Could you check a few things on this model? Use its own coordinates, in mm. Face numbers are marked on the shaded views. A direction names the side the tool comes from. Round coordinates to 2 decimals unless told otherwise and drop trailing zeros. Loops run counter-clockwise (first coordinate to the right, second up) from the corner with the lowest first, then second, coordinate; pieces in that order, holes last.
from build123d import *

# Parameters (mm, degrees)
BOSS_EXTRUDE1_DEPTH = 6.5
BOSS_EXTRUDE2_START = 6.5
SKETCH1_4_R         = 7.5
SKETCH1_4_R_2       = 1.55
BOSS_EXTRUDE2_DEPTH = 9
CUT_EXTRUDE1_DEPTH  = 15
CHAMFER1_SIZE       = 5
FILLET1_R           = 1
CUT_EXTRUDE2_DEPTH  = 3


with BuildPart() as part:
    # Sketch1 → Boss-Extrude1 (new, symmetric)
    with BuildSketch(Plane(origin=(0, 0, 0), x_dir=(1, 0, 0), z_dir=(0, 1, 0))):
        with BuildLine():
            Line((-1, 0), (0, 0))
            Line((0, 0), (0, 16))
            Line((0, 16), (-16, 16))
            ThreePointArc((-16, 16), (-17.414213562, 15.414213562), (-18, 14))
            Line((-18, 14), (-18, -14))
            ThreePointArc((-18, -14), (-10.5, -6.5), (-3, -14))
            Line((-3, -14), (-3, -2))
            ThreePointArc((-3, -2), (-2.414213562, -0.585786438), (-1, 0))
        make_face()
    extrude(amount=BOSS_EXTRUDE1_DEPTH, both=True)

    # Sketch1<4> → Boss-Extrude2 (add)
    with BuildSketch(Plane(origin=(0, 0, 0), x_dir=(1, 0, 0), z_dir=(0, 1, 0)).offset(BOSS_EXTRUDE2_START)):
        with Locations((-10.5, -14)):
            Circle(SKETCH1_4_R)
        with Locations(Location((-10.5, -14, 0), (0, 0, 270))):
            Circle(SKETCH1_4_R_2, mode=Mode.SUBTRACT)
    extrude(amount=-BOSS_EXTRUDE2_DEPTH)

    # Sketch2 → Cut-Extrude1 (cut)
    with BuildSketch(Plane(origin=(0, 0, 0), x_dir=(0, 0, -1), z_dir=(1, 0, 0))):
        with BuildLine():
            ThreePointArc((12.5, 0), (9.505604778, 4.240654932), (4.507486999, 2.837666813))
            Line((4.507486999, 2.837666813), (11.492513001, -2.837666813))
            ThreePointArc((11.492513001, -2.837666813), (12.240654932, -1.505604778), (12.5, 0))
        make_face()
        with BuildLine():
            Line((11.492513001, -2.837666813), (4.507486999, 2.837666813))
            ThreePointArc((4.507486999, 2.837666813), (5.162333187, -3.492513001), (11.492513001, -2.837666813))
        make_face()
    extrude(amount=-CUT_EXTRUDE1_DEPTH, mode=Mode.SUBTRACT)

    # Chamfer1
    # the kernel refuses this chamfer: 5 mm, written as the material it takes off along each edge
    with BuildSketch(Plane(origin=(-10.5, -6.5, 14), x_dir=(-0.003141587485879666, 0, 0.9999950652018581), z_dir=(0.9999950652018581, 0, 0.003141587485879666))) as chamfer1_piece_1_section:
        Polygon((7.5 + CHAMFER1_SIZE, 0), (7.5, -CHAMFER1_SIZE), (7.5, 0), align=None)
    chamfer1_piece_1 = revolve(axis=Axis((-10.5, -6.5, 14), (0, -1, 0)), revolution_arc=359.64, mode=Mode.PRIVATE)
    chamfer1_piece_1 = split(chamfer1_piece_1, bisect_by=Plane(origin=(-3, -4.630818152, 8.578188697), z_dir=(-1, 0, 0)), keep=Keep.TOP, mode=Mode.PRIVATE)
    chamfer1_piece_1 = split(chamfer1_piece_1, bisect_by=Plane(origin=(-19.50426243, -2.5, 8.578188697), z_dir=(0, -1, 0)), keep=Keep.TOP, mode=Mode.PRIVATE)
    add(chamfer1_piece_1, mode=Mode.SUBTRACT)
    with BuildSketch(Plane(origin=(-10.5, -6.5, 14), x_dir=(-0.003141587485879666, 0, 0.9999950652018581), z_dir=(0.9999950652018581, 0, 0.003141587485879666))) as chamfer1_piece_2_section:
        Polygon((7.5 + CHAMFER1_SIZE, 0), (7.5, -CHAMFER1_SIZE), (7.5, 0), align=None)
    chamfer1_piece_2 = revolve(axis=Axis((-10.5, -6.5, 14), (0, -1, 0)), revolution_arc=359.64, mode=Mode.PRIVATE)
    chamfer1_piece_2 = split(chamfer1_piece_2, bisect_by=Plane(origin=(-3, -5.259335852, 13.999999991), z_dir=(1, 0, 0)), keep=Keep.TOP, mode=Mode.PRIVATE)
    chamfer1_piece_2 = split(chamfer1_piece_2, bisect_by=Plane(origin=(-1.451043379, -2.5, 13.999999991), z_dir=(0, -1, 0)), keep=Keep.TOP, mode=Mode.PRIVATE)
    add(chamfer1_piece_2, mode=Mode.SUBTRACT)

    # Fillet1
    # the kernel refuses this fillet: 1 mm, written as the material it takes off along each edge
    with BuildSketch(Plane(origin=(2.5, -6.5, -16), x_dir=(0, 0, 1), z_dir=(-1, 0, 0)), Plane(origin=(2.5, 6.5, -16), x_dir=(0, -1, 0), z_dir=(-1, 0, 0))) as fillet1_piece_1:
        with BuildLine():
            CenterArc((FILLET1_R, FILLET1_R), FILLET1_R, 180, 90)
            Line((0, FILLET1_R), (0, 0))
            Line((0, 0), (FILLET1_R, 0))
        make_face()
    extrude(amount=21, mode=Mode.SUBTRACT)

    # Sketch3 → Cut-Extrude2 (cut)
    with BuildSketch(Plane.XZ.offset(2.5)):
        with BuildLine():
            Line((-7.477661315, 13.923391433), (-8.005921993, 15.110168858))
            Line((-8.005921993, 15.110168858), (-8.53418267, 16.296946283))
            ThreePointArc((-8.53418267, 16.296946283), (-8.690530367, 16.49005478), (-8.922485692, 16.579117797))
            Line((-8.922485692, 16.579117797), (-10.21439543, 16.715019342))
            Line((-10.21439543, 16.715019342), (-11.506305167, 16.850920888))
            ThreePointArc((-11.506305167, 16.850920888), (-11.75171588, 16.81207406), (-11.944824377, 16.655726364))
            Line((-11.944824377, 16.655726364), (-12.708473437, 15.604850484))
            Line((-12.708473437, 15.604850484), (-13.472122497, 14.553974605))
            ThreePointArc((-13.472122497, 14.553974605), (-13.561185513, 14.32201928), (-13.522338685, 14.076608567))
            Line((-13.522338685, 14.076608567), (-12.994078007, 12.889831142))
            Line((-12.994078007, 12.889831142), (-12.46581733, 11.703053717))
            ThreePointArc((-12.46581733, 11.703053717), (-12.309469633, 11.50994522), (-12.077514308, 11.420882203))
            Line((-12.077514308, 11.420882203), (-10.78560457, 11.284980658))
            Line((-10.78560457, 11.284980658), (-9.493694833, 11.149079112))
            ThreePointArc((-9.493694833, 11.149079112), (-9.24828412, 11.18792594), (-9.055175623, 11.344273636))
            Line((-9.055175623, 11.344273636), (-8.291526563, 12.395149516))
            Line((-8.291526563, 12.395149516), (-7.527877503, 13.446025395))
            ThreePointArc((-7.527877503, 13.446025395), (-7.438814487, 13.67798072), (-7.477661315, 13.923391433))
        make_face()
    extrude(amount=-CUT_EXTRUDE2_DEPTH, mode=Mode.SUBTRACT)


solid = part.part
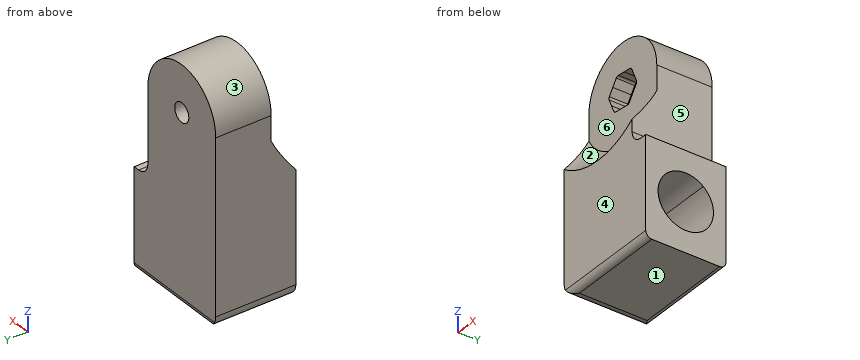
Item 1: If I drill on line 1 along X through (y, z) = (2.65, 14); line 2 along Z through (x, y) = (-1, 0); line 3 along Y through (x, z) = (-5.75, 7), over which ranges is the centre line in solid material (lowest first)?
Results list:
line 1: x = -18 to -12.05, -8.95 to -3
line 2: z = -16 to -12.5, -3.5 to 0
line 3: y = -2.5 to 6.5
Item 2: If we section it at B-B, the plane z = -10: Please give me the cut outline in (x, y).
Results list:
outline: (-18, -6.5) - (0, -6.5) - (0, -4.03) - (-15, -4.03) - (-15, 4.03) - (0, 4.03) - (0, 6.5) - (-18, 6.5) - close
Item 3: We'd pull the mould along X, two halves only. Please class the marked faces 1, 2 and 3: released by +X, released by -X, zero draft, split by the parting line, or undercut.
Results list:
face 1: zero draft
face 2: undercut
face 3: split by the parting line
Item 4: If we section it at D-D, the plane y = 1.5: Please give me the cut outline in (x, z), then the cut area to 3 significant figures.
Results list:
outline: (-18, -14) arc R2 ccw to (-16, -16) - (0, -16) - (0, -12.24) - (-15, -12.24) - (-15, -3.76) - (0, -3.76) - (0, 0) - (-1, 0) arc R2 cw to (-3, 2) - (-3, 14) arc R7.5 ccw to (-18, 14) - close; hole circle Ø3.1 at (-10.5, 14)
area: 452 mm2
Item 5: If we section it at A-A, the plane y = 4: Please give me the cut outline in (x, z).
Results list:
outline: (-18, -14) arc R2 ccw to (-16, -16) - (0, -16) - (0, -10.06) - (-15, -10.06) - (-15, -5.94) - (0, -5.94) - (0, 0) - (-1, 0) arc R2 cw to (-3, 2) - (-3, 14) arc R7.5 ccw to (-18, 14) - close; hole circle Ø3.1 at (-10.5, 14)
Item 6: Will these pins go through, and if not, where does the flat tip stop? pin 1 (4 mm diameter, centred on x = -10.5, z = 14, fed in from -Y); pin 2 (2 mm diameter, centred on y = 1, z = 12, fed in from +X); pin 3 (4.5 mm diameter, centred on y = -0.5, z = -10, fed in from +X).
Results list:
pin 1: stops at y = 0.5
pin 2: stops at x = -3
pin 3: stops at x = -15
Item 7: For the marked faces 4, 5 and 6, which set-ups out of +Z, -Z, +X, -X, +Y, -Y let a thin tool reach every point of the face, with its end or its side?
Results list:
face 4: +Z, -Z, +X, -X, -Y
face 5: +Z, +X, +Y, -Y
face 6: +Z, -Y
Item 8: If we section it at C-C, the plane y = -3.75: Please give me the cut outline in (x, z), then the cut area to 3 significant figures.
Results list:
outline: (-18, -14) arc R2 ccw to (-16, -16) - (0, -16) - (0, -10.49) - (-15, -10.49) - (-15, -5.51) - (0, -5.51) - (0, 0) - (-1, 0) arc R2 cw to (-3, 2) - (-3, 7.77) arc R9.75 cw to (-18, 7.77) - close
area: 293 mm2
